from build123d import *

# Parameters (mm, degrees)
F1_DEPTH = 63.5
F2_DEPTH = 25.4
F3_DEPTH = 7.9375
F5_R     = 6.35


with BuildPart() as f1:
    # F0 (on Front) → F1 (new body, symmetric)
    with BuildSketch(Plane.XZ):
        Polygon((-41.275, 9.525), (-41.275, -9.525), (41.275, -9.525), (41.275, 9.525), (22.225, 9.525), align=None)
    extrude(amount=F1_DEPTH, both=True)

    # F0 (on Front) → F2 (join, symmetric)
    with BuildSketch(Plane.XZ):
        with BuildLine():
            Line((22.225, 9.525), (41.275, 9.525))
            Line((41.275, 9.525), (41.275, 27.0354386152))
            ThreePointArc((41.275, 27.0354386152), (46.3048805337, 38.6284972609), (58.2071585843, 42.8752))
            Line((58.2071585843, 42.8752), (60.325, 42.8752))
            Line((60.325, 42.8752), (60.325, 61.9252))
            Line((60.325, 61.9252), (58.718494664, 61.9252))
            add(Edge.make_bspline(
                [(52.1296454234, 61.5977253585), (54.3011827008, 61.7480105937), (56.4978888968, 61.8577059663), (58.718494664, 61.9252)],
                knots=[108.0061657204, 108.0061657204, 108.0061657204, 108.0061657204, 112.8914520022, 112.8914520022, 112.8914520022, 112.8914520022], degree=3))
            ThreePointArc((52.1296454234, 61.5977253585), (30.7389084986, 49.8873503669), (22.225, 27.0354386152))
            Line((22.225, 27.0354386152), (22.225, 9.525))
        make_face()
        Polygon((85.725, 61.9252), (60.325, 61.9252), (60.325, 42.8752), (85.725, 42.8752), (85.725, 52.3875), align=None)
    extrude(amount=F2_DEPTH, both=True)

    # F0 (on Front) → F3 (join, symmetric)
    with BuildSketch(Plane.XZ):
        with BuildLine():
            add(Edge.make_bspline(
                [(-41.275, 9.525), (-31.5868860998, 35.1128955364), (4.1202962213, 58.2751499583), (52.1296454234, 61.5977253585)],
                knots=[0, 0, 0, 0, 108.0061657204, 108.0061657204, 108.0061657204, 108.0061657204], degree=3))
            Line((-41.275, 9.525), (22.225, 9.525))
            Line((22.225, 9.525), (22.225, 27.0354386152))
            ThreePointArc((22.225, 27.0354386152), (30.7389084986, 49.8873503669), (52.1296454234, 61.5977253585))
        make_face()
    extrude(amount=F3_DEPTH, both=True)

    # F0 (on Front) → F4 (revolve)
    with BuildSketch(Plane.XZ):
        Polygon((85.725, 66.675), (85.725, 61.9252), (85.725, 52.3875), (85.725, 42.8752), (85.725, 38.1), (111.125, 38.1), (111.125, 66.675), align=None)
    revolve(axis=Axis((85.725, 0, 52.3875), (0, 0, -1)))

    # F5
    f5_edges = [f1.edges().sort_by_distance(p)[0] for p in [
        (-41.275, -63.5, 0),
        (41.275, -63.5, 0),
        (41.275, 63.5, 0),
        (-41.275, 63.5, 0),
    ]]
    fillet(f5_edges, radius=F5_R)


solid = f1.part
Work out the finished part from the listing and answer in its coordinate system (mm). A direction names the side the tool comes from. Coordinates: 2 decimals unless noted, no trailing zeros. Loops run counter-clockwise (first coordinate to the right, second up) from the corner with the lowest first, then second, coordinate; pieces in that order, holes last. Notation, with made-up numbers: M 21.25,27.5 L 41.25,27.5 A10 ccw 41.25,44.5 Z; hole C 75.25,76.5 d8. An arc over 180 degrees is marked long. Answer in a Markdown table with one row per item. Add a question column.
1. Find section B-B, the plane x = 80. Write down the section's boundary in (y, z) (3 decimals).
2. Find section A-A, the plane z = 2. Write down the section's boundary in (x, y) (3 decimals), then the cut area to 3 significant figures.
3. Find section C-C, the plane y = -50.5. Write down the section's boundary in (x, z) (3 decimals).
4. A tool of negligible diameter and unlimited length cuts with its end or side. For faces 1 (the flat face through (41.275, -1, 4)), 2 (the flat face through (-4, 7.938, 30)), 3 (the flat face through (46, 25.4, 42)), 4 (the flat face through (22.225, -17, 18)), from which of +Z, -Z, +X, -X, +Y, -Y can it reach the whole face along a straight path? Write none if from no direction.
5. Flat-ended cylindrical pins translate along their axes: P1, Ø5, axis at y = 13, z = 18, coming from the -X side (3 decimals); P2, Ø8, axis at x = 87.5, y = 20.5, coming from the -Z side; P3, Ø8, axis at y = 20, z = 2.5, coming from the +X side (3 decimals); P4, Ø15.5, axis at x = 49.5, z = 25, coming from the -Y side. Find the tip coordinate at first contact, or state that the pin passes through.
6. The mould has two halves that part along X. Classify faces 5 (the cylindrical face through (-39.464, 61.59, -0.133)), 6 (the flat face through (86, 0, 38.1)), 7 (the flat face through (60, 0, 42.875)): pulls with the +X half, pulls with the -X half, needs draft (parallel to the pull), parting line crosses it, or undercut.
7. Consider L1, parallel to X at y = -26, z = 6 (3 decimals); L2, parallel to X at y = 19, z = 40.5; L3, parallel to Z at x = -29, y = -47 (3 decimals). Determine where each line is inside the solid, lowest interval first.
Reported:
| question | item | result |
|---|---|---|
| 1 | outline | M -25.4,42.875 L -24.746,42.875 L -24.746,38.1 L 24.746,38.1 L 24.746,42.875 L 25.4,42.875 L 25.4,61.925 L 24.746,61.925 L 24.746,66.675 L -24.746,66.675 L -24.746,61.925 L -25.4,61.925 Z |
| 2 | outline | M -41.275,-57.15 A6.35 ccw -34.925,-63.5 L 34.925,-63.5 A6.35 ccw 41.275,-57.15 L 41.275,57.15 A6.35 ccw 34.925,63.5 L -34.925,63.5 A6.35 ccw -41.275,57.15 Z |
| 2 | area | 10,400 mm^2 |
| 3 | outline | M -41.275,-9.525 L 41.275,-9.525 L 41.275,9.525 L -41.275,9.525 Z |
| 4 | face 1 | -Z, +X, +Y, -Y |
| 4 | face 2 | +Z, -X, +Y |
| 4 | face 3 | +Z, +X, -X, +Y |
| 4 | face 4 | +Z, -X, -Y |
| 5 | P1 | stops at x = 22.225 |
| 5 | P2 | stops at z = 38.1 |
| 5 | P3 | stops at x = 41.275 |
| 5 | P4 | passes through |
| 6 | face 5 | pulls with the -X half |
| 6 | face 6 | needs draft |
| 6 | face 7 | undercut |
| 7 | L1 | x = -41.275 to 41.275 |
| 7 | L2 | x = 24.92 to 48.74, 68.87 to 102.58 |
| 7 | L3 | z = -9.525 to 9.525 |
